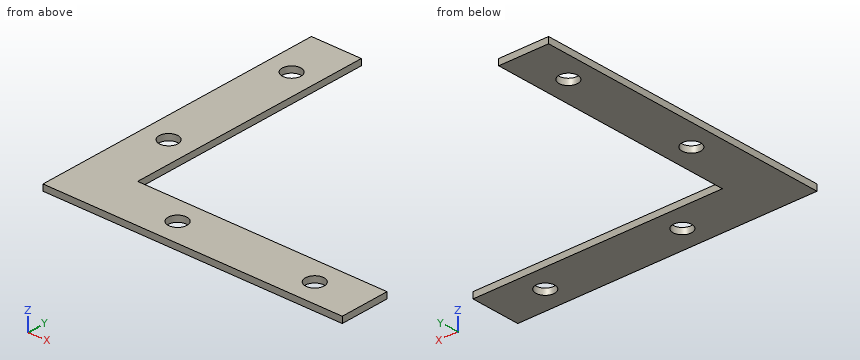
```python
from build123d import *

# Parameters (mm, degrees)
SKETCH1_R           = 2.38125
BOSS_EXTRUDE1_DEPTH = 1.5875


with BuildPart() as part:
    # Sketch1 → Boss-Extrude1 (new body)
    with BuildSketch(Plane.XY):
        Polygon((0, 0), (0, 76.2), (12.7, 76.2), (12.7, 12.7), (76.2, 12.7), (76.2, 0), align=None)
        with Locations((63.5, 6.35)):
            Circle(SKETCH1_R, mode=Mode.SUBTRACT)
        with Locations((28.575, 6.35)):
            Circle(SKETCH1_R, mode=Mode.SUBTRACT)
        with Locations(Location((6.35, 63.5, 0), (0, 0, 180))):
            Circle(SKETCH1_R, mode=Mode.SUBTRACT)
        with Locations(Location((6.35, 28.575, 0), (0, 0, 180))):
            Circle(SKETCH1_R, mode=Mode.SUBTRACT)
    extrude(amount=BOSS_EXTRUDE1_DEPTH)


solid = part.part
```
Check sheet for the modelled part. Datum: model origin and axes. Units: mm. Round coordinates to 2 decimals unless told otherwise and drop trailing zeros. Order: outer loops, then holes, each group sorted by start corner. A loop starts at its lowest first (then second) coordinate and runs counter-clockwise, first axis right, second up. Notation, with made-up numbers: (1, 24) -> (56, 24) arc R7 cw to (56, 34) -> close; hole circle Ø9 at (12.5, 61). An arc over 180 degrees is marked (long way). One line per item, written item: value. Start each with the question number.
Q1. Thickness scan on line 1 (Y direction, x = 6.35, z = 1.05); line 2 (Y direction, x = 63.5, z = 1.25); line 3 (Y direction, x = 70.5, z = 1.15). Record the ranges inside material, lowest first.
Q2. Cross-section at A-A (y = 63.5). Record the boundary of the cut face in (x, z).
Q3. Cross-section at D-D (z = 1.2). Give the number of separate pieces and of enclosed holes in the cut face, and give its area (3 significant figures).
Q4. Cross-section at B-B (x = 6.35). Record the boundary of the cut face in (y, z), and give its area (3 significant figures).
Completed:
1. line 1: y = 0 to 26.19, 30.96 to 61.12, 65.88 to 76.2
1. line 2: y = 0 to 3.97, 8.73 to 12.7
1. line 3: y = 0 to 12.7
2. outline: (0, 0) -> (3.97, 0) -> (3.97, 1.59) -> (0, 1.59) -> close; (8.73, 0) -> (12.7, 0) -> (12.7, 1.59) -> (8.73, 1.59) -> close
3. separate pieces: 1
3. enclosed holes: 4
3. area: 1,700 mm²
4. outline: (0, 0) -> (26.19, 0) -> (26.19, 1.59) -> (0, 1.59) -> close; (30.96, 0) -> (61.12, 0) -> (61.12, 1.59) -> (30.96, 1.59) -> close; (65.88, 0) -> (76.2, 0) -> (76.2, 1.59) -> (65.88, 1.59) -> close
4. area: 106 mm²
